```python
from build123d import *

# Parameters (mm, degrees)
F0_W      = 355.6
F0_H      = 50.8
F1_DEPTH  = 25.4
F3_DEPTH  = 6.35
F4_R      = 4.7625
F5_DEPTH  = 25.4
F6_R      = 12.7
F6_R_2    = 9.525
F7_DEPTH  = 25.4
F8_W      = 25.4
F8_H      = 50.8
F9_DEPTH  = 152.4
F10_W     = 50.8
F10_H     = 25.4
F11_DEPTH = 152.4
F12_R     = 12.7
F12_R_2   = 9.525
F13_DEPTH = 2.54
F14_R     = 9.525
F15_DEPTH = 25.4
F16_W     = 50.8
F16_H     = 101.6
F17_DEPTH = 6.35
F18_R     = 6.35
F19_DEPTH = 25.4
F20_W     = 50.8
F20_H     = 6.35
F21_DEPTH = 3.175


with BuildPart() as f1:
    # F0 (on Top) → F1 (new body)
    with BuildSketch(Plane.XY):
        with Locations((177.8, 11.79309)):
            Rectangle(F0_W, F0_H)
    extrude(amount=F1_DEPTH)

    # F2 (on Top) → F3 (join)
    with BuildSketch(Plane.XY):
        Polygon((355.6, 37.19309), (304.8, 37.19309), (304.8, -13.60691), (355.6, -64.40691), (406.4, -64.40691), (406.4, 37.19309), align=None)
    extrude(amount=-F3_DEPTH)

    # F4 (on face) → F5 (cut)
    with BuildSketch(Plane.XY):
        with Locations((381, -43.76941)):
            Circle(F4_R)
        with Locations((381, 7.03059)):
            Circle(F4_R)
    extrude(amount=-F5_DEPTH, mode=Mode.SUBTRACT)

    # F6 (on face) → F7 (join)
    with BuildSketch(Plane.XY.offset(25.4)):
        with Locations((76.2, 11.79309)):
            Circle(F6_R)
        with Locations((76.2, 11.79309)):
            Circle(F6_R_2, mode=Mode.SUBTRACT)
    extrude(amount=F7_DEPTH)

    # F8 (on face) → F9 (join)
    with BuildSketch(Plane.XY.offset(25.4)):
        with Locations((12.7, 11.79309)):
            Rectangle(F8_W, F8_H)
    extrude(amount=F9_DEPTH)

    # F10 (on face) → F11 (join)
    with BuildSketch(Plane(origin=(0, 0, 0), x_dir=(0, -1, 0), z_dir=(-1, 0, 0))):
        with Locations((-11.79309, 101.6)):
            Rectangle(F10_W, F10_H)
    extrude(amount=F11_DEPTH)

    # F12 (on face) → F13 (join)
    with BuildSketch(Plane(origin=(0, 0, 0), x_dir=(0, -1, 0), z_dir=(-1, 0, 0))):
        with Locations((-16.909977, 149.112195)):
            Circle(F12_R)
        with Locations((-16.909977, 149.112195)):
            Circle(F12_R_2, mode=Mode.SUBTRACT)
    extrude(amount=F13_DEPTH)

    # F14 (on face) → F15 (cut)
    with BuildSketch(Plane(origin=(0, 0, 0), x_dir=(0, -1, 0), z_dir=(-1, 0, 0))):
        with Locations((-16.909977, 149.112195)):
            Circle(F14_R)
    extrude(amount=-F15_DEPTH, mode=Mode.SUBTRACT)

    # F16 (on face) → F17 (join)
    with BuildSketch(Plane(origin=(0, 0, 88.9), x_dir=(1, 0, 0), z_dir=(0, 0, -1))):
        with Locations((-127, -37.19309)):
            Rectangle(F16_W, F16_H)
    extrude(amount=F17_DEPTH)

    # F18 (on face) → F19 (cut)
    with BuildSketch(Plane.XY.offset(88.9)):
        with Locations((-124.950424, 62.59309)):
            Circle(F18_R)
    extrude(amount=-F19_DEPTH, mode=Mode.SUBTRACT)

    # F20 (on face) → F21 (join)
    with BuildSketch(Plane.YZ.offset(-101.6)):
        Polygon((37.19309, 88.9), (87.99309, 88.9), (37.19309, 114.3), align=None)
        with Locations((62.59309, 85.725)):
            Rectangle(F20_W, F20_H)
    extrude(amount=-F21_DEPTH)

    # F22: F1 across face


with BuildPart() as f1_1:
    add(f1.part)
    add(f1.part.mirror(Plane(origin=(-152.4, 20.259757, 96.308333), x_dir=(0, -1, 0), z_dir=(-1, 0, 0))))


solid = f1_1.part
```
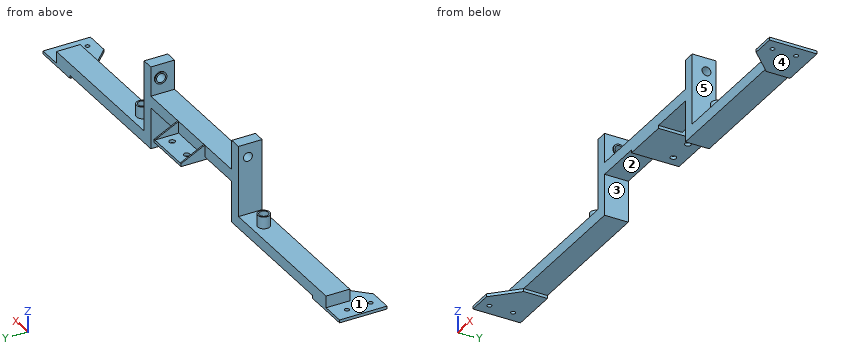
Build history of the part. All positions in model axes, mm. Face numbers are marked on the shaded views. A direction names the side the tool comes from. Give positions to 0.01 mm unless a question says otherwise; leave off trailing zeros. Order: outer loops, then holes, each group sorted by start corner. A loop starts at its lowest first (then second) coordinate and runs counter-clockwise, first axis right, second up. Notation, with made-up numbers: M 43,-36.75 L 77,-36.75 A27 ccw 77,-1.75 Z; hole C 14,85.5 d3. An arc over 180 degrees is marked long. Return JSON: item names as keys, results as strings.
Q1. Band-saw the part on B-B (y = -24.5). Give the cut face in (x, z).
Answer list:
{"outline": "M -711.2,-6.35 L -620.49,-6.35 L -620.49,0 L -711.2,0 Z; M 315.69,-6.35 L 406.4,-6.35 L 406.4,0 L 315.69,0 Z"}
Q2. Band-saw the part on A-A (x = 76.2). Give the cut face in (y, z).
Answer list:
{"outline": "M -13.61,0 L 37.19,0 L 37.19,25.4 L 24.49,25.4 L 24.49,50.8 L 21.32,50.8 L 21.32,25.4 L 2.27,25.4 L 2.27,50.8 L -0.91,50.8 L -0.91,25.4 L -13.61,25.4 Z"}
Q3. 3-axis set-ups, long thin cutter, end or side, ignore diameter. For the marked faces 3, 4 and 5: which of +Z, -Z, +X, -X, +Y, -Y reach the whole face in a straight line?
Answer list:
{"face 3": "-Z, +Y, -Y", "face 4": "-Z, +X, -X, +Y, -Y", "face 5": "+Z, +Y, -Y"}
Q4. Wall check: probe 1 along X at (y, z) = (6.5, 85.5); probe 2 along Y at (x, z) = (381, -2.75); probe 3 along X at (y, z) = (61, 86). Give the ranges that are in metal, low to high. Write a range as from..to.
Answer list:
{"probe 1": "x = -330.2..-304.8, -203.2..-101.6, 0..25.4", "probe 2": "y = -64.41..-48.53, -39.01..2.27, 11.79..37.19", "probe 3": "x = -203.2..-186, -173.7..-131.1, -118.8..-101.6"}
Q5. Band-saw the part on C-C (x = -315.5). Give the cut face in (y, z) (3 decimals), then the cut area to 3 significant figures.
Answer list:
{"outline": "M -13.607,0 L 37.193,0 L 37.193,177.8 L -13.607,177.8 Z; hole C 16.91,149.112 d19.05", "area": "8,750 mm^2"}
Q6. Band-saw the part on D-D (x = 241). Give the cut face in (y, z).
Answer list:
{"outline": "M -13.61,0 L 37.19,0 L 37.19,25.4 L -13.61,25.4 Z"}
Q7. Flat gauge pins, fed straight in: pin 1 (20.5 mm diameter, centred on y = 62.5, z = 101.5, fed in from +X); pin 2 (1 mm diameter, centred on y = -13, z = 60.5, fed in from -X); pin 3 (1.5 mm diameter, centred on x = -306.5, z = 129.5, fed in from +Y). Where does each tip first touch, or does it go through?
Answer list:
{"pin 1": "stops at x = -101.6", "pin 2": "stops at x = -330.2", "pin 3": "stops at y = 37.19"}
Q8. Two-plate mould, pull along X, no slides. Class the marked faces 1 and 2: pulls with the +X half, pulls with the -X half, needs draft (parallel to the pull), parting line crosses it, or undercut.
Answer list:
{"face 1": "needs draft", "face 2": "undercut"}
